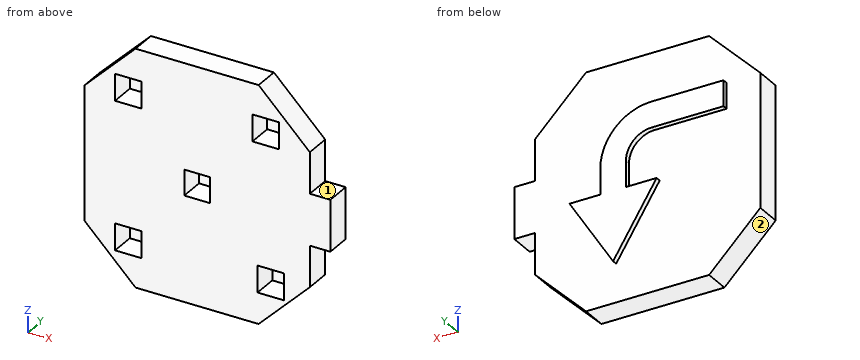
```python
from build123d import *

# Parameters (mm, degrees)
BOSS_EXTRU_1_DEPTH      = 5
BOSS_EXTRU_2_DEPTH      = 1
ESQUISSE3_W             = 5.2
ESQUISSE3_H             = 5.2
ESQUISSE3_W_2           = 5
ESQUISSE3_H_2           = 5
ENL_V_MAT_EXTRU_1_DEPTH = 4.8
CONG_1_R                = 10
CONG_2_R                = 5


with BuildPart() as part:
    # Esquisse1 → Boss.-Extru.1 (new body)
    with BuildSketch(Plane(origin=(0, 0, 0), x_dir=(1, 0, 0), z_dir=(0, 1, 0))):
        Polygon((22, 13), (12.003020456, 23), (-12.003020456, 23), (-22, 13), (-22, -13), (-12.003020456, -23), (12.003020456, -23), (22, -13), (22, -5), (26, -5), (26, 5), (22, 5), align=None)
    extrude(amount=BOSS_EXTRU_1_DEPTH)

    # Esquisse2 → Boss.-Extru.2 (add)
    with BuildSketch(Plane(origin=(0, 5, 0), x_dir=(1, 0, 0), z_dir=(0, 1, 0))):
        Polygon((-15.409608561, -8), (3.631850655, -8), (3.631850655, 2), (-2.368149345, 2), (6.131850655, 15.555441712), (14.631850655, 2), (8.631850655, 2), (8.631850655, -13), (-15.409608561, -13), align=None)
    extrude(amount=BOSS_EXTRU_2_DEPTH)

    # Esquisse3 → Enlèv. mat.-Extru.1 (cut)
    with BuildSketch(Plane.XZ):
        with Locations((-13.4, 14.4)):
            Rectangle(ESQUISSE3_W, ESQUISSE3_H)
        with Locations((-13.4, -14.4)):
            Rectangle(ESQUISSE3_W, ESQUISSE3_H)
        with Locations((14.4, -14.4)):
            Rectangle(ESQUISSE3_W, ESQUISSE3_H)
        with Locations((13.4, 14.4)):
            Rectangle(ESQUISSE3_W, ESQUISSE3_H)
        Rectangle(ESQUISSE3_W_2, ESQUISSE3_H_2)
    extrude(amount=-ENL_V_MAT_EXTRU_1_DEPTH, mode=Mode.SUBTRACT)

    # Congé1
    cong_1_edges = [part.edges().sort_by_distance(p)[0] for p in [
        (8.631850655, 5.5, 13),
    ]]
    fillet(cong_1_edges, radius=CONG_1_R)

    # Congé2
    cong_2_edges = [part.edges().sort_by_distance(p)[0] for p in [
        (3.631850655, 5.5, 8),
    ]]
    fillet(cong_2_edges, radius=CONG_2_R)


solid = part.part
```
Work out the finished part from the listing and answer in its coordinate system (mm). Face numbers are marked on the shaded views. A direction names the side the tool comes from. Round coordinates to 2 decimals unless told otherwise and drop trailing zeros. Order: outer loops, then holes, each group sorted by start corner. A loop starts at its lowest first (then second) coordinate and runs counter-clockwise, first axis right, second up.
Q1. Given pin 1 Ø1 at (y, z) = (5, 15) entering from -X; pin 2 Ø4 at (x, z) = (-14, 13) entering from -Y; pin 3 Ø2 at (x, y) = (19, 1) entering from +Z; pin 4 Ø3 at (x, z) = (8.5, -16) entering from +Y, each flat-ended and moving along its own axis, determine where each tip first touches the part or whether it passes through.
Solution:
pin 1: stops at x = -20.5
pin 2: stops at y = 0
pin 3: stops at z = 17
pin 4: stops at y = 5
Q2. A cutting plane is placed at D-D, the plane z = 15.5. Determine the outline of the cut face in (x, y).
Solution:
outline: (-19.5, 0) - (-16, 0) - (-16, 4.8) - (-10.8, 4.8) - (-10.8, 0) - (10.8, 0) - (10.8, 4.8) - (16, 4.8) - (16, 0) - (19.5, 0) - (19.5, 5) - (-19.5, 5) - close
Q3. A cutting plane is placed at C-C, the plane z = 6. Determine the outline of the cut face in (x, y).
Solution:
outline: (-22, 0) - (22, 0) - (22, 5) - (8.17, 5) - (8.17, 6) - (2.63, 6) - (2.63, 5) - (-22, 5) - close
Q4. Find the intervals of material crossed by line 1 along Z through (x, y) = (13, 2.05); line 2 along Z through (x, y) = (-11.5, 3.1); line 3 along X through (y, z) = (4.2, 0.5), in increasing order.
Solution:
line 1: z = -22 to -17, -11.8 to 11.8, 17 to 22
line 2: z = -23 to -17, -11.8 to 11.8, 17 to 23
line 3: x = -22 to -2.5, 2.5 to 26
Q5. A cutting plane is placed at B-B, the plane x = -8. Determine the outline of the cut face in (y, z).
Solution:
outline: (0, -23) - (5, -23) - (5, 8) - (6, 8) - (6, 13) - (5, 13) - (5, 23) - (0, 23) - close
Q6. A tool of negligible diameter and unlimited length cuts with its end or side. For the marked faces 1 and 2, from which of +Z, -Z, +X, -X, +Y, -Y can it reach the whole face along a straight path? Write none if from no direction.
Solution:
face 1: +Z, +X, +Y, -Y
face 2: -Z, -X, +Y, -Y
Q7. A cutting plane is placed at A-A, the plane y = 3.8. Count the separate pieces of the cut face and the enclosed holes in it, then the cut area to 3 significant figures.
Solution:
separate pieces: 1
enclosed holes: 5
area: 1,730 mm2
